Geometry check sheet. Reference: the model listing, model coordinates, mm. Face numbers are marked on the shaded views. A direction names the side the tool comes from. Give positions to 0.01 mm unless a question says otherwise; leave off trailing zeros. Write each loop counter-clockwise with the first axis right and the second up, starting at its lowest first coordinate (ties: lowest second). Pieces come first, ordered by that corner, then holes. Notation, with made-up numbers: (54.25, 8) - (103.25, 8) arc R19 ccw to (103.25, 41) - close; hole circle Ø7 at (85.5, 2.25). An arc over 180 degrees is marked (long way). Write item = value, one per line. Start each with the question number.
(1) Depth check by flat-ended pin: pin 1 Ø1.5 at (x, y) = (-9, 11) entering from +Z. Enter the tip coordinate at first touch or a pass-through.
(2) Draft check along X on the marked faces 3, 4, 5 and 6. Enter one of: pulls with the +X half, pulls with the -X half, needs draft (parallel to the pull), parting line crosses it, or undercut.
(3) Section check C-C, the plane x = -30. Enter the section's corners in (y, z).
(4) Access from +Z, -Z, +X, -X, +Y, -Y to the whole of each face (thin tool, end or side, straight path). Record for the marked faces 1 and 2.
(5) Section check A-A, the plane z = 51.5. Enter the section's corners in (x, y).
(6) Thickness scan on L1, parallel to Y at x = -17, z = 9; L2, parallel to X at y = -22, z = 22.5; L3, parallel to Z at x = -26, y = 9.5. Record the ranges inside material, lowest first.
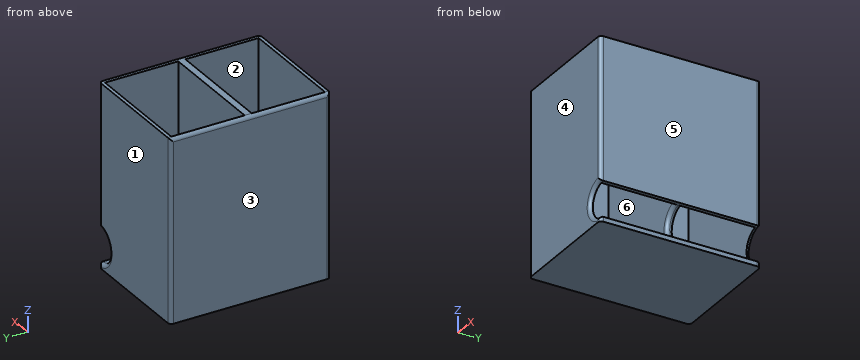
```python
from build123d import *

# Parameters (mm, degrees)
F1_DEPTH = 34
F2_T     = -1.5
F3_DEPTH = 2
F6_R     = 1.49999


# Not quite as in the source:
# - a fillet or chamfer is up to 0.001 mm smaller than in the source, because OpenCascade refuses the exact size


with BuildPart() as f1:
    # F0 (on Front) → F1 (new body)
    with BuildSketch(Plane.XZ):
        with BuildLine():
            Line((0, 75), (-50, 75))
            Line((-50, 75), (-50, 0))
            Line((-50, 0), (0, 0))
            ThreePointArc((0, 0), (-7.5, 7.5), (0, 15))
            Line((0, 15), (0, 75))
        make_face()
    extrude(amount=F1_DEPTH)

    # F2
    f2_openings = [f1.faces().sort_by_distance(p)[0] for p in [
        (-25, -17, 75),
        (-7.5, -17, 7.5),
    ]]
    offset(amount=F2_T, openings=f2_openings)

    # F3 (add): a face of the model
    f3_faces = [f1.faces().sort_by_distance(p)[0] for p in [
        (-25, -17, 0),
    ]]
    extrude(f3_faces, amount=F3_DEPTH)


with BuildPart() as f4_1:
    # F4: instance of F1
    add(f1.part.mirror(Plane(origin=(-25.5124575843, 0, 37.1811815231), x_dir=(-1, 0, 0), z_dir=(0, 1, 0))))


with BuildPart() as f1_1:
    add(f1.part)

    # F5: union F4_1
    add(f4_1.part)

    # F6 (radius 1.5 in the source; OpenCascade refuses exactly that, so slightly less here)
    f6_edges = [f1_1.edges().sort_by_distance(p)[0] for p in [
        (0, -34, 45),
        (-50, -34, 36.5),
        (-50, 34, 36.5),
        (0, 34, -1),
        (0, -34, -1),
        (-50, 0, 75),
        (0, 34, 45),
        (-7.5, 34, 7.5),
        (-7.317473, 1.5, 9.144564),
        (-7.317473, -1.5, 9.144564),
        (-7.5, -34, 7.5),
    ]]
    fillet(f6_edges, radius=F6_R)


solid = f1_1.part
```
Model answer:
q1.pin_1 = 1.5
q2.face_3 = pulls with the -X half
q2.face_4 = needs draft
q2.face_5 = pulls with the +X half
q2.face_6 = undercut
q3.outline = (-34, -2) - (34, -2) - (34, 75) - (32.5, 75) - (32.5, 1.5) - (1.5, 1.5) - (1.5, 75) - (-1.5, 75) - (-1.5, 1.5) - (-32.5, 1.5) - (-32.5, 75) - (-34, 75) - close
q4.face_1 = +Z, -Z, +X, -X, +Y
q4.face_2 = +Z
q5.outline = (-50, -32.5) arc R1.5 ccw to (-48.5, -34) - (-1.5, -34) arc R1.5 ccw to (0, -32.5) - (0, 32.5) arc R1.5 ccw to (-1.5, 34) - (-48.5, 34) arc R1.5 ccw to (-50, 32.5) - close; hole (-48.5, -32.5) - (-1.5, -32.5) - (-1.5, -1.5) - (-48.5, -1.5) - close; hole (-48.5, 1.5) - (-1.5, 1.5) - (-1.5, 32.5) - (-48.5, 32.5) - close
q6.L1 = -34 to -32.5, -1.5 to 1.5, 32.5 to 34
q6.L2 = -50 to -48.5, -1.5 to 0
q6.L3 = -2 to 1.5
